```python
from build123d import *

# Parameters (mm, degrees)
BOSS_EXTRUDE1_DEPTH = 10
BOSS_EXTRUDE2_START = 35
SKETCH2_R           = 2.5
BOSS_EXTRUDE2_DEPTH = 7
LPATTERN1_COUNT     = 3
LPATTERN1_PITCH     = 35
SHELL1_T            = -3
SKETCH3_W           = 8
SKETCH3_H           = 20
CUT_EXTRUDE1_DEPTH  = 20
BOSS_EXTRUDE3_START = -3
SKETCH5_R           = 2.5
BOSS_EXTRUDE3_DEPTH = 3
LPATTERN2_COUNT     = 2
LPATTERN2_PITCH     = 31
SKETCH6_W           = 28
SKETCH6_H           = 14
CUT_EXTRUDE2_DEPTH  = 3


with BuildPart() as part:
    # Sketch1 → Boss-Extrude1 (new body, symmetric)
    with BuildSketch(Plane(origin=(0, 0, 0), x_dir=(1, 0, 0), z_dir=(0, 1, 0))):
        Polygon((-45, 0), (45, 0), (30, -100), (-30, -100), align=None)
    extrude(amount=BOSS_EXTRUDE1_DEPTH, both=True)

    # Sketch2 → Boss-Extrude2 (add, symmetric)
    with BuildSketch(Plane(origin=(0, 0, 0), x_dir=(0, 0, -1), z_dir=(1, 0, 0)).offset(BOSS_EXTRUDE2_START)):
        with BuildLine():
            Line((0, 10), (10, 10))
            ThreePointArc((10, 10), (20, 0), (10, -10))
            Line((10, -10), (0, -10))
            Line((0, -10), (0, 10))
        make_face()
        with Locations((10, 0)):
            Circle(SKETCH2_R, mode=Mode.SUBTRACT)
    boss_extrude2 = extrude(amount=BOSS_EXTRUDE2_DEPTH, both=True)

    # LPattern1: Boss-Extrude2 ×3
    with Locations(*[(-i * LPATTERN1_PITCH, 0, 0) for i in range(1, LPATTERN1_COUNT)]):
        add(boss_extrude2)

    # Shell1
    shell1_openings = [part.faces().sort_by_distance(p)[0] for p in [
        (0, 0, 100),
    ]]
    offset(amount=SHELL1_T, openings=shell1_openings, kind=Kind.INTERSECTION)

    # Sketch3 → Cut-Extrude1 (cut)
    with BuildSketch(Plane.XY):
        with Locations((35, 0)):
            Rectangle(SKETCH3_W, SKETCH3_H)
        Rectangle(SKETCH3_W, SKETCH3_H)
        with Locations((-35, 0)):
            Rectangle(SKETCH3_W, SKETCH3_H)
    extrude(amount=-CUT_EXTRUDE1_DEPTH, mode=Mode.SUBTRACT)

    # Sketch5 → Boss-Extrude3 (add)
    with BuildSketch(Plane(origin=(-14.009779951, 0, 93.398533007), x_dir=(0.988936353, 0, 0.148340453), z_dir=(-0.148340453, 0, 0.988936353)).offset(BOSS_EXTRUDE3_START)):
        with BuildLine():
            Line((44.502135879, 10), (54.502135879, 10))
            ThreePointArc((54.502135879, 10), (64.502135879, 0), (54.502135879, -10))
            Line((54.502135879, -10), (44.502135879, -10))
            Line((44.502135879, -10), (44.502135879, 10))
        make_face()
        with Locations((54.502135879, 0)):
            Circle(SKETCH5_R, mode=Mode.SUBTRACT)
    boss_extrude3 = extrude(amount=-BOSS_EXTRUDE3_DEPTH)

    # LPattern2: Boss-Extrude3 ×2
    with Locations(*[Vector(0.148340453, 0, -0.988936353) * (i * LPATTERN2_PITCH) for i in range(1, LPATTERN2_COUNT)]):
        add(boss_extrude3)

    # Sketch6 → Cut-Extrude2 (cut)
    with BuildSketch(Plane(origin=(44.009779951, 0, 6.601466993), x_dir=(0.148340453, 0, -0.988936353), z_dir=(0.988936353, 0, 0.148340453))):
        with Locations((-74.443421699, 0)):
            Rectangle(SKETCH6_W, SKETCH6_H)
    extrude(amount=-CUT_EXTRUDE2_DEPTH, mode=Mode.SUBTRACT)


solid = part.part
```
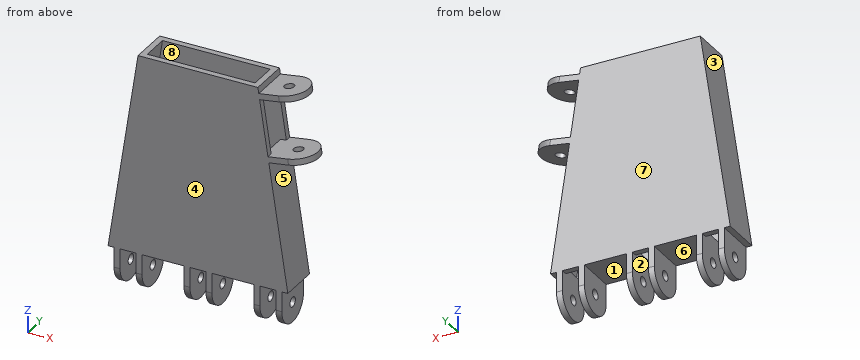
Here's how the part is built. I have some questions about the finished solid (model axes, mm). Face numbers are marked on the shaded views. A direction names the side the tool comes from. Coordinates: 2 decimals unless noted, no trailing zeros. Order: outer loops, then holes, each group sorted by start corner. A loop starts at its lowest first (then second) coordinate and runs counter-clockwise, first axis right, second up.
1) Which directions (+Z, -Z, +X, -X, +Y, -Y) give clear straight access to the entire face, cutting with the end or side of a thin tool? Please do the marked faces 5, 6, 7 and 8.
2) We'd pull the mould along X, two halves only. Please class the marked faces 1, 2, 3 and 4: +X half, -X half, draft (parallel to the pull), parting line (faces both ways), or undercut.
3) Imagine slicing it at D-D on x = 23.5. List the corners of the cut face in (y, z) for me.
4) Imagine slicing it at A-A on x = -0.5. List the corners of the cut face in (y, z) for me.
5) Will these pins go through, and if not, where does the flat tip stop? pin 1 (2 mm diameter, centred on x = 35.5, y = -5.5, fed in from +Z); pin 2 (1.5 mm diameter, centred on x = 43, y = -5, fed in from -Z); pin 3 (1.3 mm diameter, centred on x = 40.5, y = 1.5, fed in from +Z); pin 4 (3 mm diameter, centred on y = 0, z = -10, fed in from -X).
6) Imagine slicing it at C-C on z = 41. List the corners of the cut face in (x, y) for me.
7) Imagine slicing it at B-B on z = -5.5. List the corners of the cut face in (x, y) for me, and give its area (3 significant figures).
8) I need wall thicknesses on line 1 (X direction, y = 6, z = -13); line 2 (Y direction, x = 12, z = 43.5); line 3 (Z direction, x = 29.9, y = 0). Which ranges of each line are inside material? Lowest first, please.
Response values:
1. face 5: +X, +Y, -Y
1. face 6: -Z, +Y, -Y
1. face 7: +Z, -Z, +X, -X, +Y
1. face 8: none
2. face 1: undercut
2. face 2: undercut
2. face 3: -X half
2. face 4: draft
3. outline: (-10, 0) - (10, 0) - (10, 100) - (7, 100) - (7, 3) - (-7, 3) - (-7, 100) - (-10, 100) - close
4. outline: (-10, 0) - (-7, 0) - (-7, 100) - (-10, 100) - close; (7, 0) - (10, 0) - (10, 100) - (7, 100) - close
5. pin 1: stops at z = 97.94
5. pin 2: stops at z = 0
5. pin 3: stops at z = 67.29
5. pin 4: passes through
6. outline: (-38.85, -10) - (38.85, -10) - (38.85, 10) - (-38.85, 10) - close; hole (-35.82, -7) - (35.82, -7) - (35.82, 7) - (-35.82, 7) - close
7. outline: (-42, -10) - (-39, -10) - (-39, 10) - (-42, 10) - close; (-31, -10) - (-28, -10) - (-28, 10) - (-31, 10) - close; (-7, -10) - (-4, -10) - (-4, 10) - (-7, 10) - close; (4, -10) - (7, -10) - (7, 10) - (4, 10) - close; (28, -10) - (31, -10) - (31, 10) - (28, 10) - close; (39, -10) - (42, -10) - (42, 10) - (39, 10) - close
7. area: 360 mm2
8. line 1: x = -42 to -39, -31 to -28, -7 to -4, 4 to 7, 28 to 31, 39 to 42
8. line 2: y = -10 to -7, 7 to 10
8. line 3: z = -20 to -12.5, -7.5 to 3, 93.92 to 100
